Input: dimensioned drawing with shaded views. Units: mm. Origin: part minimum x, y, z. Round coordinates to 2 decimals unless told otherwise and drop trailing zeros. Loops run counter-clockwise (first coordinate to the right, second up) from the corner with the lowest first, then second, coordinate; pieces in that order, holes last. Notation, with made-up numbers: (-39.5, 16.25) - (-27.5, 16.25) arc R23 cw to (-27.5, 26.25) - close; hole circle Ø5 at (84, 54.25). An arc over 180 degrees is marked (long way). Answer as a JSON object with one key per item and string values. Group by question number.
Item 1: Line query: line 1 (Y direction, x = 50, z = 4.5); line 2 (Y direction, x = 50, z = 36.5); line 3 (X direction, y = 44, z = 13). Output: solid intervals per line, ascending.
Item 2: Draft query along X for the marked faces 1, 2, 3 and 4. Return one class per face: released by +X, released by -X, zero draft, split by the parting line, or undercut.
Item 3: Section C-C (z = 25.5). Return the cut outline in (x, y), plus the area to 3 significant figures.
Item 4: Section D-D (y = 67). Return the cut outline in (x, z), plus the area to 3 significant figures.
Item 5: Section A-A (y = 50). Return the cut outline in (x, z), plus the area to 3 significant figures.
Item 6: First-contact query: pin 1 (3 mm diameter, centred on x = 11, y = 22, fed in from +Z); pin 2 (1 mm diameter, centred on x = 64.5, z = 11.5, fed in from -Y); pin 3 (10 mm diameter, centred on x = 63, z = 13, fed in from +Y). Flat tips, straight axial feed; report the tip coordinate or a pass-through.
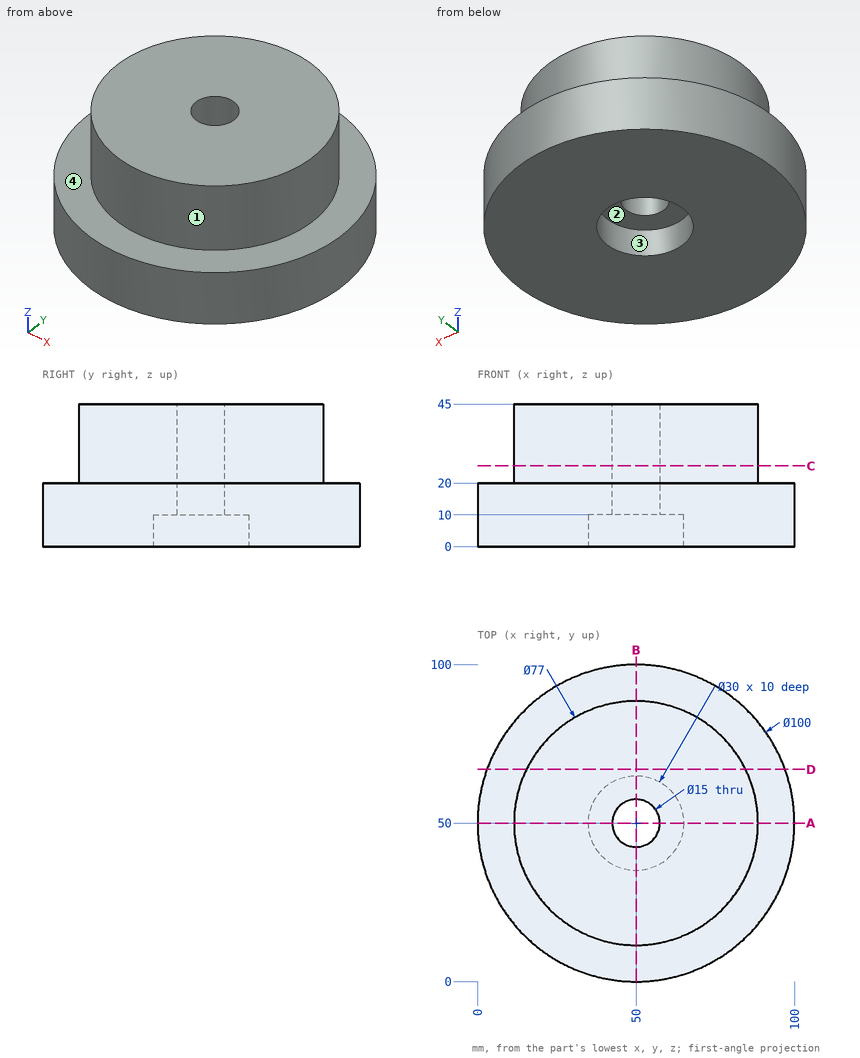
Values:
{
 "1": {"line 1": "y = 0 to 35, 65 to 100", "line 2": "y = 11.5 to 42.5, 57.5 to 88.5", "line 3": "x = 0.36 to 45.5, 54.5 to 99.64"},
 "2": {"face 1": "split by the parting line", "face 2": "undercut", "face 3": "undercut", "face 4": "zero draft"},
 "3": {"outline": "circle Ø77 at (50, 50); hole circle Ø15 at (50, 50)", "area": "4,480 mm^2"},
 "4": {"outline": "(2.98, 0) - (97.02, 0) - (97.02, 20) - (84.54, 20) - (84.54, 45) - (15.46, 45) - (15.46, 20) - (2.98, 20) - close", "area": "3,610 mm^2"},
 "5": {"outline": "(0, 0) - (35, 0) - (35, 10) - (42.5, 10) - (42.5, 45) - (11.5, 45) - (11.5, 20) - (0, 20) - close; (57.5, 10) - (65, 10) - (65, 0) - (100, 0) - (100, 20) - (88.5, 20) - (88.5, 45) - (57.5, 45) - close", "area": "3,100 mm^2"},
 "6": {"pin 1": "stops at z = 20", "pin 2": "stops at y = 2", "pin 3": "stops at y = 99.36"}
}
